For this review, take the finished solid that the model builds, in its own axes (mm). A direction names the side the tool comes from. Give positions to 0.01 mm unless a question says otherwise; leave off trailing zeros. Order: outer loops, then holes, each group sorted by start corner. A loop starts at its lowest first (then second) coordinate and runs counter-clockwise, first axis right, second up. Notation, with made-up numbers: (58, -36.5) -> (95, -36.5) arc R23 cw to (95, -8.5) -> close; hole circle Ø1 at (78.5, 86). An arc over 180 degrees is marked (long way). One line per item, written item: value. Start each with the question number.
from build123d import *

# Parameters (mm, degrees)
CROQUIS1_W              = 13
CROQUIS1_H              = 8
CROQUIS1_W_2            = 8
CROQUIS1_H_2            = 21
CROQUIS1_R              = 1.5
SALIENTE_EXTRUIR1_DEPTH = 4
CROQUIS2_R              = 2.85
CORTAR_EXTRUIR1_DEPTH   = 1.65
CROQUIS3_W              = 4
CROQUIS3_H              = 3
CORTAR_EXTRUIR2_DEPTH   = 13


with BuildPart() as part:
    # Croquis1 → Saliente-Extruir1 (new body)
    # profile 1 of 2: a face of its own
    with BuildSketch(Plane.XY):
        with Locations((11.5, -79)):
            Rectangle(CROQUIS1_W, CROQUIS1_H)
    # profile 2 of 2: a face of its own
    with BuildSketch(Plane.XY):
        with Locations((1, -72.5)):
            Rectangle(CROQUIS1_W_2, CROQUIS1_H_2)
        with Locations((1, -66.715045403)):
            Circle(CROQUIS1_R, mode=Mode.SUBTRACT)
        with Locations((1, -79)):
            Circle(CROQUIS1_R, mode=Mode.SUBTRACT)
    extrude(amount=SALIENTE_EXTRUIR1_DEPTH)

    # Croquis2 → Cortar-Extruir1 (cut)
    with BuildSketch(Plane.XY.offset(4)):
        with Locations((1, -79)):
            Circle(CROQUIS2_R)
        with Locations((1, -66.715045403)):
            Circle(CROQUIS2_R)
    extrude(amount=-CORTAR_EXTRUIR1_DEPTH, mode=Mode.SUBTRACT)

    # Croquis3 → Cortar-Extruir2 (cut)
    with BuildSketch(Plane(origin=(18, 0, 0), x_dir=(0, 0, -1), z_dir=(1, 0, 0))):
        with Locations((-2, -76.5)):
            Rectangle(CROQUIS3_W, CROQUIS3_H)
    extrude(amount=-CORTAR_EXTRUIR2_DEPTH, mode=Mode.SUBTRACT)


solid = part.part
Q1. Mouldability with a two-part tool opening along X and no side actions: class faces 4 (the flat face through (3, -75, 0)), 5 (the cylindrical face through (1.806, -77.735, 1.159)), 6 (the flat face through (5, -70, 2)) as pulls with the +X half, pulls with the -X half, needs draft (parallel to the pull), parting line crosses it, or undercut.
Q2. For faces 1 (the flat face through (7, -83, 2)), 2 (the flat face through (2.2, -80.2, 2.35)), 3 (the flat face through (12, -78, 2)), list the 3-axis set-ups (+Z, -Z, +X, -X, +Y, -Y) from which the entire face can be reached by the end or side of a thin tool; tool diameter is ignored.
Q3. For pin 1 Ø1 at (y, z) = (-70, 1) entering from +X; pin 2 Ø3.5 at (x, y) = (1, -66.72) entering from +Z, all flat-tipped, find the tip position at first contact; note any pin that passes through.
Q4. Take a section at C-C (z = 3.75). State the section outline as (x, y) points, and give its area (3 significant figures).
Q5. Take a section at B-B (x = 1). State the section outline as (y, z) points, and give its area (3 significant figures).
Q6. For line 1 along Y through (x, z) = (1, 3.25); line 2 along Y through (x, z) = (1, 1.5); line 3 along X through (y, z) = (-79, 1), list the stretches that pass through material, from the lowest coordinate up.
Q7. Take a section at A-A (y = -79). State the section outline as (x, z) points, and give its area (3 significant figures).
Q8. Take a section at D-D (x = 3.25). State the section outline as (y, z) points, and give its area (3 significant figures).
Answers below:
1. face 4: needs draft
1. face 5: undercut
1. face 6: pulls with the +X half
2. face 1: +Z, -Z, +X, -X, -Y
2. face 2: +Z
2. face 3: +Z, -Z, +X, +Y
3. pin 1: stops at x = 5
3. pin 2: stops at z = 2.35
4. outline: (-3, -83) -> (18, -83) -> (18, -78) -> (5, -78) -> (5, -62) -> (-3, -62) -> close; hole circle Ø5.7 at (1, -79); hole circle Ø5.7 at (1, -66.72)
4. area: 182 mm²
5. outline: (-83, 0) -> (-80.5, 0) -> (-80.5, 2.35) -> (-81.85, 2.35) -> (-81.85, 4) -> (-83, 4) -> close; (-77.5, 0) -> (-68.22, 0) -> (-68.22, 2.35) -> (-69.57, 2.35) -> (-69.57, 4) -> (-76.15, 4) -> (-76.15, 2.35) -> (-77.5, 2.35) -> close; (-65.22, 0) -> (-62, 0) -> (-62, 4) -> (-63.87, 4) -> (-63.87, 2.35) -> (-65.22, 2.35) -> close
5. area: 51.1 mm²
6. line 1: y = -83 to -81.85, -76.15 to -69.57, -63.87 to -62
6. line 2: y = -83 to -80.5, -77.5 to -68.22, -65.22 to -62
6. line 3: x = -3 to -0.5, 2.5 to 18
7. outline: (-3, 0) -> (-0.5, 0) -> (-0.5, 2.35) -> (-1.85, 2.35) -> (-1.85, 4) -> (-3, 4) -> close; (2.5, 0) -> (18, 0) -> (18, 4) -> (3.85, 4) -> (3.85, 2.35) -> (2.5, 2.35) -> close
7. area: 67.5 mm²
8. outline: (-83, 0) -> (-62, 0) -> (-62, 4) -> (-64.97, 4) -> (-64.97, 2.35) -> (-68.46, 2.35) -> (-68.46, 4) -> (-77.25, 4) -> (-77.25, 2.35) -> (-80.75, 2.35) -> (-80.75, 4) -> (-83, 4) -> close
8. area: 72.5 mm²
